```python
from build123d import *

# Parameters (mm, degrees)
SKETCH4_R          = 1.25
CUT_EXTRUDE1_DEPTH = 25.129857072


with BuildPart() as part:
    # Sketch2 → Revolve1 (revolve)
    with BuildSketch(Plane.XY, mode=Mode.PRIVATE) as revolve1_sk:
        with BuildLine():
            Line((-8.5, 13.3), (8.5, 13.3))
            Line((8.5, 13.3), (8.5, 12.75))
            Line((8.5, 12.75), (11.225, 12.75))
            Line((11.225, 12.75), (11.5, 13.025))
            Line((11.5, 13.025), (11.5, 14.725))
            ThreePointArc((11.5, 14.725), (11.419454365, 14.919454365), (11.225, 15))
            Line((11.225, 15), (2, 15))
            ThreePointArc((2, 15), (0, 14.5), (-2, 15))
            Line((-2, 15), (-11.225, 15))
            ThreePointArc((-11.225, 15), (-11.419454365, 14.919454365), (-11.5, 14.725))
            Line((-11.5, 14.725), (-11.5, 13.025))
            Line((-11.5, 13.025), (-11.225, 12.75))
            Line((-11.225, 12.75), (-8.5, 12.75))
            Line((-8.5, 12.75), (-8.5, 13.3))
        make_face()
    revolve(revolve1_sk.sketch.rotate(Axis((-11.5, 0, 0), (1, 0, 0)), 180), axis=Axis((-11.5, 0, 0), (1, 0, 0)))

    # Sketch4 → Cut-Extrude1 (cut, through all)
    with BuildSketch(Plane(origin=(0, 0, 0), x_dir=(1, 0, 0), z_dir=(0, 1, 0))):
        with Locations(Location((0, 0, 0), (0, 0, 90))):
            Circle(SKETCH4_R)
    extrude(amount=CUT_EXTRUDE1_DEPTH, mode=Mode.SUBTRACT)


solid = part.part
```
Verification items for the finished model (mm, model axes). A direction names the side the tool comes from. Coordinates: 2 decimals unless noted, no trailing zeros. Loops run counter-clockwise (first coordinate to the right, second up) from the corner with the lowest first, then second, coordinate; pieces in that order, holes last. Notation, with made-up numbers: (84.25, -26.75) -> (97.25, -26.75) arc R20 cw to (97.25, 11.25) -> close; hole circle Ø2 at (63, 7). An arc over 180 degrees is marked (long way). Put each result on its own line as item: value.
1. Section check D-D, the plane x = 3. Record the boundary of the cut face in (y, z).
Result set:
outline: circle Ø30 at (0, 0); hole circle Ø26.6 at (0, 0)
2. Gauge pin test, flat ends, axial feed: P1, Ø3, axis at x = 0, z = 0, coming from the -Y side; P2, Ø1, axis at x = 1.5, y = -3.5, coming from the +Z side; P3, Ø12, axis at x = -6.5, y = 9, coming from the -Z side. Record the tip position at first contact, or that the pin passes through.
Result set:
P1: stops at y = -14.77
P2: stops at z = 14.61
P3: stops at z = -14.7
3. Mould release check, pull along X, two halves, no side actions. Record for faces 1 (the face through (9.882, 2.764, 12.447)), 2 (the face through (0.119, -12.286, 5.094)), 3 (the face through (11.5, 9, 10)): pulls with the +X half, pulls with the -X half, needs draft (parallel to the pull), parting line crosses it, or undercut.
Result set:
face 1: needs draft
face 2: undercut
face 3: pulls with the +X half
4. Section check A-A, the plane z = 0. Give the number of separate pieces and of enclosed holes in the cut face, then the cut area to 3 significant figures.
Result set:
separate pieces: 3
enclosed holes: 0
area: 78.7 mm^2
5. Thickness scan on line 1 (Z direction, x = 9.25, y = 0); line 2 (Y direction, x = 5.5, z = 0.5); line 3 (Z direction, x = -9.75, y = 11). Record the ranges inside material, lowest first.
Result set:
line 1: z = -15 to -12.75, 12.75 to 15
line 2: y = -14.99 to -13.29, 13.29 to 14.99
line 3: z = -10.2 to -6.45, 6.45 to 10.2
6. Section check B-B, the plane y = 0. Record the boundary of the cut face in (x, z) (3 decimals), then the cut area to 3 significant figures.
Result set:
outline: (-11.5, -14.725) arc R0.275 ccw to (-11.225, -15) -> (-2, -15) arc R4.25 cw to (2, -15) -> (11.225, -15) arc R0.275 ccw to (11.5, -14.725) -> (11.5, -13.025) -> (11.225, -12.75) -> (8.5, -12.75) -> (8.5, -13.3) -> (-8.5, -13.3) -> (-8.5, -12.75) -> (-11.225, -12.75) -> (-11.5, -13.025) -> close; (-11.5, 13.025) -> (-11.225, 12.75) -> (-8.5, 12.75) -> (-8.5, 13.3) -> (8.5, 13.3) -> (8.5, 12.75) -> (11.225, 12.75) -> (11.5, 13.025) -> (11.5, 14.725) arc R0.275 ccw to (11.225, 15) -> (2, 15) arc R4.25 cw to (-2, 15) -> (-11.225, 15) arc R0.275 ccw to (-11.5, 14.725) -> close
area: 81.9 mm^2
7. Tool access check on faces 4 (the face through (-8.5, 11, 7)), 5 (the face through (-0.38, 13.95, -1.19)), 6 (the face through (-6.68, -8.06, -12.65)). Record the directions out of +Z, -Z, +X, -X, +Y, -Y that give a thin tool (end or side, any length) a straight path to the whole face; none if there is none.
Result set:
face 4: none
face 5: +Y
face 6: +X, -X
8. Section check C-C, the plane x = -10. Record the boundary of the cut face in (y, z), then the cut area to 3 significant figures.
Result set:
outline: circle Ø30 at (0, 0); hole circle Ø25.5 at (0, 0)
area: 196 mm^2
